Here's how the part is built. I have some questions about the finished solid (model axes, mm). Face numbers are marked on the shaded views. A direction names the side the tool comes from. Give positions to 0.01 mm unless a question says otherwise; leave off trailing zeros. Write each loop counter-clockwise with the first axis right and the second up, starting at its lowest first coordinate (ties: lowest second). Pieces come first, ordered by that corner, then holes. Notation, with made-up numbers: M 49.5,61 L 79.5,61 A10 cw 79.5,74 Z; hole C 43,82 d3. An arc over 180 degrees is marked long. Use one line per item in the form item = value. Start each with the question number.
from build123d import *

# Parameters (mm, degrees)
SKETCH_1_W          = 25
SKETCH_1_H          = 36
SKETCH_1_R          = 1.65
EXTRUDE_1_DEPTH     = 5
SKETCH_2_W          = 14
SKETCH_2_H          = 20
EXTRUDE_2_DEPTH     = 25
SKETCH_3_R          = 5
CUT_EXTRUDE_1_DEPTH = 35
FILLET_1_R          = 7
FILLET_2_R          = 7
FILLET_3_R          = 7
FILLET_4_R          = 7
FILLET_5_R          = 2


with BuildPart() as part:
    # ｽｹｯﾁ1 → ﾎﾞｽ - 押し出し1 (new body)
    with BuildSketch(Plane.XY):
        with Locations((-12.5, 0)):
            Rectangle(SKETCH_1_W, SKETCH_1_H)
        with Locations((-20, 0)):
            Circle(SKETCH_1_R, mode=Mode.SUBTRACT)
    extrude(amount=EXTRUDE_1_DEPTH)

    # ｽｹｯﾁ2 → ﾎﾞｽ - 押し出し2 (add)
    with BuildSketch(Plane.XY.offset(5)):
        with Locations((-7, 0)):
            Rectangle(SKETCH_2_W, SKETCH_2_H)
    extrude(amount=EXTRUDE_2_DEPTH)

    # ｽｹｯﾁ3 → ｶｯﾄ - 押し出し1 (cut)
    with BuildSketch(Plane.XY.offset(30)):
        Circle(SKETCH_3_R)
    extrude(amount=-CUT_EXTRUDE_1_DEPTH, mode=Mode.SUBTRACT)

    # ﾌｨﾚｯﾄ1
    fillet_1_edges = [part.edges().sort_by_distance(p)[0] for p in [
        (-14, 10, 17.5),
    ]]
    fillet(fillet_1_edges, radius=FILLET_1_R)

    # ﾌｨﾚｯﾄ2
    fillet_2_edges = [part.edges().sort_by_distance(p)[0] for p in [
        (-14, -10, 17.5),
    ]]
    fillet(fillet_2_edges, radius=FILLET_2_R)

    # ﾌｨﾚｯﾄ3
    fillet_3_edges = [part.edges().sort_by_distance(p)[0] for p in [
        (-25, 18, 2.5),
    ]]
    fillet(fillet_3_edges, radius=FILLET_3_R)

    # ﾌｨﾚｯﾄ4
    fillet_4_edges = [part.edges().sort_by_distance(p)[0] for p in [
        (-25, -18, 2.5),
    ]]
    fillet(fillet_4_edges, radius=FILLET_4_R)

    # ﾌｨﾚｯﾄ5
    fillet_5_edges = [part.edges().sort_by_distance(p)[0] for p in [
        (-3.5, 10, 30),
        (-5, 0, 30),
        (-14, 0, 30),
        (-11.949747468, 7.949747468, 30),
        (-3.5, -10, 30),
        (-11.949747468, -7.949747468, 30),
    ]]
    fillet(fillet_5_edges, radius=FILLET_5_R)


solid = part.part
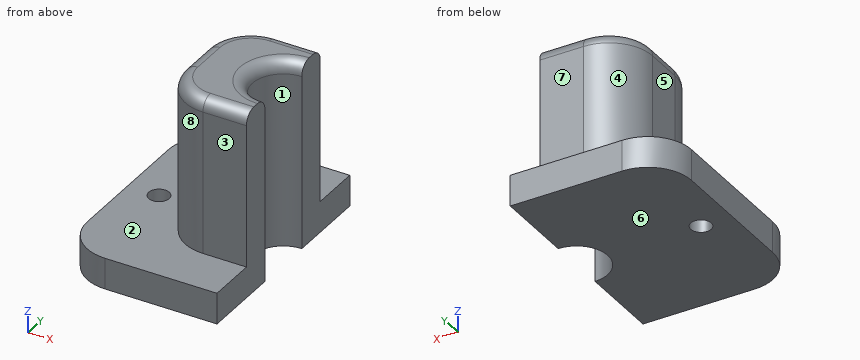
1) On a 3-axis mill with a long thin cutter (end or side, diameter ignored), from which of +Z, -Z, +X, -X, +Y, -Y can I reach the whole of each face in a straight line? I mean the marked faces 5, 6, 7 and 8. Say none if no direction works.
2) Suppose I cut it at A-A, the plane y = 0. List the corners of the cut face in (x, z) for me.
3) Suppose I cut it at B-B, the plane z = 27. List the corners of the cut face in (x, y) for me, and give its area (3 significant figures).
4) Suppose I cut it at C-C, the plane x = -20. List the corners of the cut face in (y, z) for me.
5) Will these pins go through, and if not, where does the flat tip stop? P1, Ø7.5, axis at x = -2, z = 22, coming from the +Y side; P2, Ø1.5, axis at x = -4.5, y = 0.5, coming from the +Z side; P3, Ø5, axis at x = -18, y = -10.5, coming from the +Z side; P4, Ø5, axis at y = 11.5, z = 10.5, coming from the +X side.
6) Thinking about a two-plate mould opening in Y: for the marked faces 1, 2, 3 and 4, which applies, released by +Y, released by -Y, zero draft, split by the parting line, or undercut?
7) Please list where these lines run through material, in increasing order: line 1 (Z direction, x = -15, y = -1); line 2 (Y direction, x = -20, z = 3.8); line 3 (Y direction, x = -3.75, z = 9).
8) Suppose I cut it at D-D, the plane x = -15.75. List the corners of the cut face in (y, z) for me.
Checks:
q1.face_5 = +Z, -X, +Y, -Y
q1.face_6 = -Z, +X, -X, +Y, -Y
q1.face_7 = +Z, +X, -X, +Y
q1.face_8 = +Z, -X, -Y
q2.outline = M -25,0 L -21.65,0 L -21.65,5 L -25,5 Z; M -18.35,0 L -5,0 L -5,28 A2 ccw -7,30 L -12,30 A2 ccw -14,28 L -14,5 L -18.35,5 Z
q3.outline = M -14,-3 A7 ccw -7,-10 L 0,-10 L 0,-5 A5 cw 0,5 L 0,10 L -7,10 A7 ccw -14,3 Z
q3.area = 220 mm^2
q4.outline = M -17.71,0 L -1.65,0 L -1.65,5 L -17.71,5 Z; M 1.65,0 L 17.71,0 L 17.71,5 L 1.65,5 Z
q5.P1 = 10
q5.P2 = 29.02
q5.P3 = 5
q5.P4 = 0
q6.face_1 = undercut
q6.face_2 = zero draft
q6.face_3 = released by -Y
q6.face_4 = released by +Y
q7.line_1 = 0 to 5
q7.line_2 = -17.71 to -1.65, 1.65 to 17.71
q7.line_3 = -10 to -3.31, 3.31 to 10
q8.outline = M -18,0 L 18,0 L 18,5 L -18,5 Z
